Could you check a few things on this model? Use its own coordinates, in mm. Give positions to 0.01 mm unless a question says otherwise; leave off trailing zeros. Loops run counter-clockwise (first coordinate to the right, second up) from the corner with the lowest first, then second, coordinate; pieces in that order, holes last. Notation, with made-up numbers: (66, 12.25) -> (125, 12.25) arc R20 ccw to (125, 16.25) -> close; hole circle Ø10 at (-31.75, 0.25). An arc over 180 degrees is marked (long way). Write each question's results on one line, items separated by ' | '. Start each with the question number.
Q1. If I drill on line 1 along Y through (x, z) = (-26.89, 1.1); line 2 along Y through (x, z) = (-26.89, 0.35); line 3 along X through (y, z) = (7, 0.2), over which ranges is the centre line in solid material (lowest first)?
Q2. If we section it at B-B, the plane z = 1.25: List the corners of the cut face in (x, y) for me.
Q3. If we section it at C-C, the plane x = 11: List the corners of the cut face in (y, z) for me, plus the area to 3 significant figures.
Q4. Will these pins go through, and if not, where does the flat tip stop? P1, Ø1.2, axis at x = 24.5, y = -11.5, coming from the -Z side; P2, Ø4, axis at x = -26.89, y = 7.32, coming from the +Z side; P3, Ø0.5, axis at y = -1, z = 1, coming from the -X side; P4, Ø0.5, axis at x = 24.5, z = 1, coming from the +Y side.
Q5. If we section it at A-A, the plane y = 21: List the corners of the cut face in (x, z) for me.
from build123d import *

# Parameters (mm, degrees)
F0_W           = 8.89
F0_H           = 24.64
F1_DEPTH       = 0.5
F3_DEPTH       = 1
F4_R           = 4
F6_D           = 2.5
F6_CBORE_D     = 7
F6_CBORE_DEPTH = 0.5
F7_W           = 5.5
F7_H           = 1
F8_DEPTH       = 3


with BuildPart() as f1:
    # F0 (on Top) → F1 (new body)
    with BuildSketch(Plane.XY):
        Polygon((-23, -25), (23, -25), (23, 25), (-23, 25), (-23, 12.32), (-23, -12.32), align=None)
        with Locations((-27.445, 0)):
            Rectangle(F0_W, F0_H)
    extrude(amount=F1_DEPTH)

    # F2 (on face) → F3 (join)
    with BuildSketch(Plane.XY.offset(0.5)):
        Polygon((-22.4, -24.4), (22.4, -24.4), (22.4, 24.4), (-22.4, 24.4), (-22.4, 11.72), (-31.29, 11.72), (-31.29, -11.72), (-22.4, -11.72), align=None)
    extrude(amount=F3_DEPTH)

    # F4
    f4_edges = [f1.edges().sort_by_distance(p)[0] for p in [
        (-31.89, 12.32, 0.25),
        (-31.29, 11.72, 1),
        (-23, 12.32, 0.25),
        (-22.4, 11.72, 1),
        (-31.29, -11.72, 1),
        (-31.89, -12.32, 0.25),
        (-23, -12.32, 0.25),
        (-22.4, -11.72, 1),
    ]]
    fillet(f4_edges, radius=F4_R)

    # F6 (through all)
    with Locations(Plane(origin=(0, 0, 0), x_dir=(1, 0, 0), z_dir=(0, 0, -1))):
        with Locations((-26.89, -7.32), (-26.89, 7.32)):
            CounterBoreHole(F6_D / 2, F6_CBORE_D / 2, F6_CBORE_DEPTH)

    # F7 (on face) → F8 (join)
    with BuildSketch(Plane.YZ.offset(22.4)):
        with Locations((-10.4, 1)):
            Rectangle(F7_W, F7_H)
        with Locations((10.4, 1)):
            Rectangle(F7_W, F7_H)
    extrude(amount=F8_DEPTH)


solid = f1.part
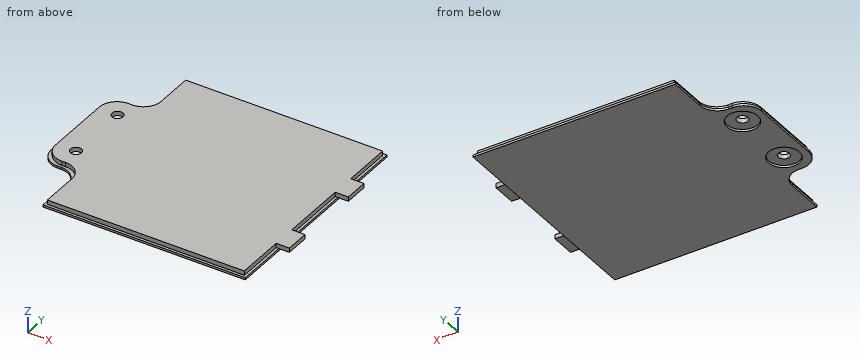
Final values:
1) line 1: y = -11.72 to -8.57, -6.07 to 6.07, 8.57 to 11.72 | line 2: y = -12.32 to -10.82, -3.82 to 3.82, 10.82 to 12.32 | line 3: x = -31.89 to -30.38, -23.4 to 23
2) outline: (-31.29, -7.72) arc R4 ccw to (-27.29, -11.72) -> (-26.4, -11.72) arc R4 cw to (-22.4, -15.72) -> (-22.4, -24.4) -> (22.4, -24.4) -> (22.4, -13.15) -> (25.4, -13.15) -> (25.4, -7.65) -> (22.4, -7.65) -> (22.4, 7.65) -> (25.4, 7.65) -> (25.4, 13.15) -> (22.4, 13.15) -> (22.4, 24.4) -> (-22.4, 24.4) -> (-22.4, 15.72) arc R4 cw to (-26.4, 11.72) -> (-27.29, 11.72) arc R4 ccw to (-31.29, 7.72) -> close; hole circle Ø2.5 at (-26.89, -7.32); hole circle Ø2.5 at (-26.89, 7.32)
3) outline: (-25, 0) -> (25, 0) -> (25, 0.5) -> (24.4, 0.5) -> (24.4, 1.5) -> (-24.4, 1.5) -> (-24.4, 0.5) -> (-25, 0.5) -> close | area: 73.8 mm²
4) P1: stops at z = 0.5 | P2: stops at z = 1.5 | P3: stops at x = -31.29 | P4: stops at y = 13.15
5) outline: (-23, 0) -> (23, 0) -> (23, 0.5) -> (22.4, 0.5) -> (22.4, 1.5) -> (-22.4, 1.5) -> (-22.4, 0.5) -> (-23, 0.5) -> close
